The model under review builds one solid part; all positions refer to its coordinate system, in mm. Give positions to 0.01 mm unless a question says otherwise; leave off trailing zeros. Loops run counter-clockwise (first coordinate to the right, second up) from the corner with the lowest first, then second, coordinate; pieces in that order, holes last. Notation, with made-up numbers: (79, 26) -> (128, 26) arc R10 cw to (128, 42) -> close; hole circle Ø5 at (42, 18). An arc over 180 degrees is marked (long way). Write each question's results on one line, items separated by ' | '. Start each with the question number.
Q1. We need section B-B (z = -19.05). Write out the cut boundary in (x, y).
Q2. We need section C-C (y = 0.95). Write out the cut boundary in (x, z).
Q3. Insertion check: pin 1 Ø12 at (x, z) = (52, -25.5) entering from -Y; pin 2 Ø10 at (x, z) = (38.1, -19.05) entering from -Y. Each pin has a flat end and moves straight along its axis. Give the tip position at first contact, or say it passes through.
Q4. We need section A-A (x = 38.1). Write out the cut boundary in (y, z).
Q5. Wall thickness on L1, parallel to X at y = 0.5, z = -19.05; L2, parallel to Z at x = 38.1, y = 1.25; L3, parallel to X at y = 1.3, z = -16.5: over which ranges is each line inside the solid? List them lowest first. Write a range as [from, to].
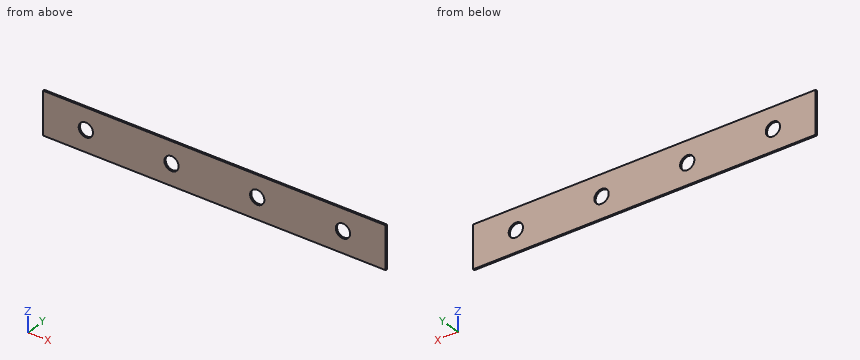
from build123d import *

# Parameters (mm, degrees)
SKETCH1_W           = 38.1
SKETCH1_H           = 1.51892
BOSS_EXTRUDE1_DEPTH = 304.8
SKETCH3_R           = 6.35
CUT_EXTRUDE1_DEPTH  = 2.51892


with BuildPart() as part:
    # Sketch1 → Boss-Extrude1 (new body)
    with BuildSketch(Plane(origin=(0, 0, 0), x_dir=(0, 0, -1), z_dir=(1, 0, 0))):
        with Locations((19.05, 0.75946)):
            Rectangle(SKETCH1_W, SKETCH1_H)
    extrude(amount=BOSS_EXTRUDE1_DEPTH)

    # Sketch3 → Cut-Extrude1 (cut, through all)
    with BuildSketch(Plane(origin=(0, 1.51892, 0), x_dir=(1, 0, 0), z_dir=(0, 1, 0))):
        with Locations((114.3, 19.05)):
            Circle(SKETCH3_R)
        with Locations((190.5, 19.05)):
            Circle(SKETCH3_R)
        with Locations((266.7, 19.05)):
            Circle(SKETCH3_R)
        with Locations((38.1, 19.05)):
            Circle(SKETCH3_R)
    extrude(amount=-CUT_EXTRUDE1_DEPTH, mode=Mode.SUBTRACT)


solid = part.part
Output:
1) outline: (0, 0) -> (31.75, 0) -> (31.75, 1.52) -> (0, 1.52) -> close; (44.45, 0) -> (107.95, 0) -> (107.95, 1.52) -> (44.45, 1.52) -> close; (120.65, 0) -> (184.15, 0) -> (184.15, 1.52) -> (120.65, 1.52) -> close; (196.85, 0) -> (260.35, 0) -> (260.35, 1.52) -> (196.85, 1.52) -> close; (273.05, 0) -> (304.8, 0) -> (304.8, 1.52) -> (273.05, 1.52) -> close
2) outline: (0, -38.1) -> (304.8, -38.1) -> (304.8, 0) -> (0, 0) -> close; hole circle Ø12.7 at (38.1, -19.05); hole circle Ø12.7 at (114.3, -19.05); hole circle Ø12.7 at (190.5, -19.05); hole circle Ø12.7 at (266.7, -19.05)
3) pin 1: y = 0 | pin 2: through
4) outline: (0, -38.1) -> (1.52, -38.1) -> (1.52, -25.4) -> (0, -25.4) -> close; (0, -12.7) -> (1.52, -12.7) -> (1.52, 0) -> (0, 0) -> close
5) L1: [0, 31.75], [44.45, 107.95], [120.65, 184.15], [196.85, 260.35], [273.05, 304.8] | L2: [-38.1, -25.4], [-12.7, 0] | L3: [0, 32.28], [43.92, 108.48], [120.12, 184.68], [196.32, 260.88], [272.52, 304.8]
